Autodesk Inventor part; units mm, degrees
ref_plane "YZ Plane" through (0, 0, 0) normal (1, 0, 0) x (0, 1, 0)
ref_plane "XZ Plane" through (0, 0, 0) normal (0, 1, 0) x (-1, 0, 0)
ref_plane "XY Plane" through (0, 0, 0) normal (0, 0, 1) x (1, 0, 0)
sketch "Sketch1" plane through (0, 0, 0) normal (0, 1, 0) x (-1, 0, 0)
  circle A0 centre (0, 0) radius 10
  dimension "d0" = 20
extrude "Extrusion1" add sketch "Sketch1" along normal blind 1.8
sketch "Sketch3" plane through (0, 1.8, 0) normal (0, 1, 0) x (1, 0, 0)
  circle A0 centre (0, 0) radius 10
  circle A1 centre (0, 0) radius 3.5
  circle A2 centre (0, 0) radius 2.5
  dimension "d3" = 7
  dimension "d4" = 5
extrude "Extrusion2" add sketch "Sketch3" along normal blind 2.4 contours A1
sketch "Sketch4" plane through (0, 0, 0) normal (0, -1, 0) x (1, 0, 0)
  circle A0 centre (0, 0) radius 10
  line L0 (0, 0) -> (6.3, 0)
  circle A1 centre (6.3, 0) radius 1.5
  dimension "d7" = 6.3
  dimension "d8" = 3
extrude "Extrusion3" cut sketch "Sketch4" against normal blind 2.4 contours A1
sketch "Sketch5" plane through (0, 0, 0) normal (0, -1, 0) x (1, 0, 0)
  circle A0 centre (0, 0) radius 10
  line L0 (0, 0) -> (-6.3, 0)
  circle A1 centre (-6.3, 0) radius 1.5
  dimension "d11" = 6.3
  dimension "d12" = 3
extrude "Extrusion4" cut sketch "Sketch5" against normal blind 2 contours A1
sketch "Sketch6" plane through (0, 0, 0) normal (0, -1, 0) x (1, 0, 0)
  circle A0 centre (-6.3, 0) radius 1.5
  circle A1 centre (6.3, 0) radius 1.5
extrude "Extrusion5" add sketch "Sketch6" against normal blind 1.8
sketch "Sketch7" plane through (0, 0, 0) normal (0, -1, 0) x (1, 0, 0)
  circle A0 centre (0, 0) radius 10
extrude "Extrusion6" add sketch "Sketch7" along normal blind 2
sketch "Sketch8" plane through (0, -2, 0) normal (0, -1, 0) x (1, 0, 0)
  circle A0 centre (0, 0) radius 10
  circle A1 centre (0, 0) radius 4
  circle A2 centre (0, 0) radius 2
  dimension "d19" = 8
  dimension "d20" = 4
extrude "Extrusion7" add sketch "Sketch8" along normal blind 4.5 contours A1
properties part number "otaceni_packy_microservo"
Source: CAD feature listing. Evaluate the final solid. Frame: model axes, mm. A direction names the side the tool comes from. Give positions to 0.01 mm unless a question says otherwise; leave off trailing zeros. Loops run counter-clockwise (first coordinate to the right, second up) from the corner with the lowest first, then second, coordinate; pieces in that order, holes last. Notation, with made-up numbers: (55, 63) -> (97, 63) arc R20 cw to (97, 67) -> close; hole circle Ø8 at (52, 69). An arc over 180 degrees is marked (long way). Use a Markdown table: item, result. Add a question column.
1) First-contact query: pin 1 (1.5 mm diameter, centred on x = -0.5, z = -0.5, fed in from +Y); pin 2 (2 mm diameter, centred on x = -3, y = 1.5, fed in from +Z); pin 3 (1.2 mm diameter, centred on x = 0.5, z = -1, fed in from -Y). Flat tips, straight axial feed; report the tip coordinate or a pass-through.
2) Pull-direction query (X, two-part tool) for faces 1 (the face through (0, -2, 0)), 2 (the face through (-2, -6.5, -1)), 3 (the face through (3.233, 2.983, -1.341)); classes: +X half, -X half, draft (parallel to the pull), parting line (faces both ways), or undercut.
3) Section query A-A, the plane z = 0. Return the cut outline in (x, y).
4) Section query D-D, the plane x = -8. Return the cut outline in (y, z), then the cut area to 3 significant figures.
5) Section query B-B, the plane x = 0. Return the cut outline in (y, z).
6) Section query C-C, the plane y = -5.25. Return the cut outline in (x, z), then the cut area to 3 significant figures.
7) Line query: line 1 along X through (y, z) = (3, 0); line 2 along Z through (x, y) = (0, -4.7). Output: solid intervals per line, ascending. Write a range as [from, to].
8) Reachability of faces 4 (the face through (0, -4, 2)), 5 (the face through (-4, 1.8, 0)), 6 (the face through (2, 4.2, 2)) from +Z, -Z, +X, -X, +Y, -Y: full face, straight path, thin tool, end or side. Return the list, or none.
Numbers:
| question | item | result |
|---|---|---|
| 1 | pin 1 | stops at y = 1.8 |
| 1 | pin 2 | stops at z = 9.8 |
| 1 | pin 3 | stops at y = -2 |
| 2 | face 1 | undercut |
| 2 | face 2 | draft |
| 2 | face 3 | parting line |
| 3 | outline | (-10, -2) -> (-4, -2) -> (-4, -6.5) -> (-2, -6.5) -> (-2, -2) -> (2, -2) -> (2, -6.5) -> (4, -6.5) -> (4, -2) -> (10, -2) -> (10, 1.8) -> (3.5, 1.8) -> (3.5, 4.2) -> (2.5, 4.2) -> (2.5, 1.8) -> (-2.5, 1.8) -> (-2.5, 4.2) -> (-3.5, 4.2) -> (-3.5, 1.8) -> (-10, 1.8) -> close |
| 4 | outline | (-2, -6) -> (1.8, -6) -> (1.8, 6) -> (-2, 6) -> close |
| 4 | area | 45.6 mm2 |
| 5 | outline | (-6.5, -4) -> (-2, -4) -> (-2, -10) -> (1.8, -10) -> (1.8, -3.5) -> (4.2, -3.5) -> (4.2, -2.5) -> (1.8, -2.5) -> (1.8, 2.5) -> (4.2, 2.5) -> (4.2, 3.5) -> (1.8, 3.5) -> (1.8, 10) -> (-2, 10) -> (-2, 4) -> (-6.5, 4) -> (-6.5, 2) -> (-2, 2) -> (-2, -2) -> (-6.5, -2) -> close |
| 6 | outline | circle Ø8 at (0, 0); hole circle Ø4 at (0, 0) |
| 6 | area | 37.7 mm2 |
| 7 | line 1 | x = [-3.5, -2.5], [2.5, 3.5] |
| 7 | line 2 | z = [-4, -2], [2, 4] |
| 8 | face 4 | -Y |
| 8 | face 5 | +Y |
| 8 | face 6 | +Z, -Z, +X, -X, +Y |
